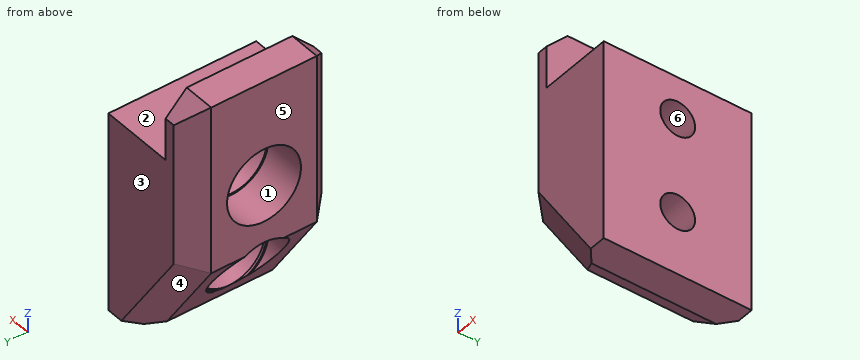
```python
from build123d import *

# Parameters (mm, degrees)
F1_DEPTH       = 7
F2_R           = 3.5
F3_DEPTH       = 4
F4_D           = 3.3
F4_START       = 4
F4_START_2     = 4.24
F4_CSINK_D     = 6.72
F4_CSINK_ANGLE = 90
F5_T1_DEPTH    = 20.2867319519
F5_T3_DEPTH    = 26.2867319519
F5_T5_DEPTH    = 21.1033857783
F5_T7_DEPTH    = 19.707629012
F6_W           = 7
F6_H           = 6
F7_DEPTH       = 7.001
F7_DEPTH_BACK  = 7.001


# Not quite as in the source:
# - a fillet or chamfer that OpenCascade refuses, or shapes differently, is made with other operations: its cross-section is extruded or revolved along the edge and cut away or added


with BuildPart() as f1:
    # F0 (on Front) → F1 (new body, symmetric)
    with BuildSketch(Plane.XZ):
        Polygon((0, -25), (0, 0), (-10, 0), (-10, -16), (-4, -25), align=None)
    extrude(amount=F1_DEPTH, both=True)

    # F2 (on face) → F3 (cut)
    with BuildSketch(Plane(origin=(-10, 0, 0), x_dir=(0, -1, 0), z_dir=(-1, 0, 0))):
        with Locations((0, -10)):
            Circle(F2_R)
        with Locations((0, -19)):
            Circle(F2_R)
    extrude(amount=-F3_DEPTH, mode=Mode.SUBTRACT)

    # F4 (through all)
    # its depths count from where the whole tool has entered the part; down to there all is cleared
    with Locations(Plane(origin=(-10, 0, 0), x_dir=(0, -1, 0), z_dir=(-1, 0, 0))):
        with Locations((0, -19, -F4_START_2), (0, -10, -F4_START)):
            CounterSinkHole(F4_D / 2, F4_CSINK_D / 2, counter_sink_angle=F4_CSINK_ANGLE)

    # F5: chamfer of 2 on 7 edges, made by hand

    # F5_s2 → F5_t1 (cut)
    with BuildSketch(Plane.YZ.offset(-15.1433659759)):
        Polygon((-7, -2), (-5, 0), (-7, 0), align=None)
        Polygon((7, -2), (5, 0), (7, 0), align=None)
    extrude(amount=F5_T1_DEPTH, mode=Mode.SUBTRACT)

    # F5_s4 → F5_t3 (cut)
    with BuildSketch(Plane.XY.offset(-21.1433659759)):
        Polygon((-8, 7), (-10, 5), (-10, 7), align=None)
        Polygon((-8, -7), (-10, -5), (-10, -7), align=None)
    extrude(amount=F5_T3_DEPTH, mode=Mode.SUBTRACT)

    # F5_s6 → F5_t5 (cut)
    with BuildSketch(Plane(origin=(1.4546661916, 0, -2.1819992874), x_dir=(0, 1, 0), z_dir=(0.5547001962, 0, -0.8320502943))):
        Polygon((-7, -15.195706083), (-5, -17.195706083), (-7, -17.195706083), align=None)
        Polygon((7, -15.195706083), (5, -17.195706083), (7, -17.195706083), align=None)
    extrude(amount=F5_T5_DEPTH, mode=Mode.SUBTRACT)

    # F5_s8 → F5_t7 (cut)
    with BuildSketch(Plane.XZ.offset(-9.853814506)):
        Polygon((-2.929632483, -25), (-4.5937330717, -24.1094003925), (-4, -25), align=None)
    extrude(amount=F5_T7_DEPTH, mode=Mode.SUBTRACT)

    # F6 (on Front) → F7 (cut, two sides)
    with BuildSketch(Plane.XZ) as f7_sk:
        with Locations((-3.5, -3)):
            Rectangle(F6_W, F6_H)
    extrude(amount=-F7_DEPTH, mode=Mode.SUBTRACT)
    extrude(f7_sk.sketch, amount=F7_DEPTH_BACK, mode=Mode.SUBTRACT)


solid = f1.part
```
For this review, take the finished solid that the model builds, in its own axes (mm). Face numbers are marked on the shaded views. A direction names the side the tool comes from. Round coordinates to 2 decimals unless told otherwise and drop trailing zeros. Write each loop counter-clockwise with the first axis right and the second up, starting at its lowest first coordinate (ties: lowest second). Pieces come first, ordered by that corner, then holes. Notation, with made-up numbers: (10.5, 85) - (30.5, 85) arc R32 cw to (30.5, 117) - close; hole circle Ø5 at (60, -31.5). An arc over 180 degrees is marked (long way). Use CSV: the item, a comma, the result in double quotes.
1) Add section D-D on x = -5. Write out the cut boundary in (y, z).
Conclusion:
outline,"(-7, -19.89) - (-5, -23.5) - (5, -23.5) - (7, -19.89) - (7, -6) - (-7, -6) - close; hole circle Ø5.2 at (0, -19); hole circle Ø4.72 at (0, -10)"
2) Add section C-C on z = -3.75. Write out the cut boundary in (x, y).
Conclusion:
outline,"(-10, -5) - (-8, -7) - (-7, -7) - (-7, 7) - (-8, 7) - (-10, 5) - close"
3) Add section B-B on x = -9.5. Write out the cut boundary in (y, z).
Conclusion:
outline,"(-5.5, -15.85) - (-5, -16.75) - (-2.68, -16.75) arc R3.5 cw to (2.68, -16.75) - (5, -16.75) - (5.5, -15.85) - (5.5, -0.5) - (5, 0) - (-5, 0) - (-5.5, -0.5) - close; hole circle Ø7 at (0, -10)"
4) Clearance check with flat-ended pins moving along their axes: pin 1 Ø4.5 at (y, z) = (0, -10) entering from -X; pin 2 Ø7 at (y, z) = (1.5, -20) entering from -X; pin 3 Ø6.5 at (y, z) = (-3.5, -2.5) entering from +X; pin 4 Ø2 at (y, z) = (-0.5, -19) entering from -X. State where each tip first meets the part, or that it passes through.
Conclusion:
pin 1,"stops at x = -4.89"
pin 2,"stops at x = -9.54"
pin 3,"stops at x = -7"
pin 4,"passes through"
5) For the marked faces 1, 2 and 3, list the 3-axis set-ups (+Z, -Z, +X, -X, +Y, -Y) from which the entire face can be reached by the end or side of a thin tool; tool diameter is ignored.
Conclusion:
face 1,"-X"
face 2,"+Z, +X, +Y, -Y"
face 3,"+Z, -Z, +X, -X, +Y"
6) The part is to be moulded in two halves that separate along Z. For the marked faces 4, 5 and 6, say which applies: pulls with the +Z half, pulls with the -Z half, needs draft (parallel to the pull), parting line crosses it, or undercut.
Conclusion:
face 4,"pulls with the -Z half"
face 5,"needs draft"
face 6,"undercut"
7) Add section A-A on z = -10. Write out the cut boundary in (x, y).
Conclusion:
outline,"(-10, -5) - (-8, -7) - (0, -7) - (0, -1.65) - (-4.29, -1.65) - (-6, -3.36) - (-6, -3.5) - (-10, -3.5) - close; (-10, 3.5) - (-6, 3.5) - (-6, 3.36) - (-4.29, 1.65) - (0, 1.65) - (0, 7) - (-8, 7) - (-10, 5) - close"
8) Wall thickness on line 1 along Z through (x, y) = (-2.75, 0); line 2 along Z through (x, y) = (-7.2, 0); line 3 along Z through (x, y) = (-1.75, -1): over which ranges is each line inside the solid? List them lowest first. Write a range as from..to.
Conclusion:
line 1,"z = -25..-20.65, -17.35..-11.65, -8.35..-6"
line 2,"z = -15.5..-13.5, -6.5..0"
line 3,"z = -25..-20.31, -17.69..-11.31, -8.69..-6"
